The listing builds one solid part. Answer for the finished solid, in the listing's coordinates (mm). A direction names the side the tool comes from. Coordinates: 2 decimals unless noted, no trailing zeros. Order: outer loops, then holes, each group sorted by start corner. A loop starts at its lowest first (then second) coordinate and runs counter-clockwise, first axis right, second up.
```python
from build123d import *

# Parameters (mm, degrees)
SKETCH_W        = 40
SKETCH_H        = 70
SKETCH_R        = 5.5
SKETCH_W_2      = 16
SKETCH_H_2      = 21.5
PAD_DEPTH       = 2
SKETCH001_W     = 5.6
SKETCH001_H     = 5.6
SKETCH001_W_2   = 16
SKETCH001_H_2   = 21.5
PAD001_DEPTH    = 6.5
SKETCH002_R     = 1.625
PAD002_DEPTH    = 2.5
SKETCH003_W     = 16.000008
SKETCH003_H     = 1
SKETCH003_W_2   = 18
POCKET_DEPTH    = 1.5
SKETCH004_W     = 5.3
SKETCH004_H     = 4.3
POCKET001_DEPTH = 2.001
SKETCH005_R     = 1.6
SKETCH005_W     = 8.4
SKETCH005_H     = 1
PAD003_DEPTH    = 1.75
SKETCH006_W     = 36
SKETCH006_H     = 66
SKETCH006_W_2   = 34.4
SKETCH006_H_2   = 64.4
PAD004_DEPTH    = 2.5


with BuildPart() as part:
    # Sketch → Pad (new body)
    with BuildSketch(Plane.XY):
        with Locations((0, -2.25)):
            Rectangle(SKETCH_W, SKETCH_H)
        with Locations((0, 20.75)):
            Circle(SKETCH_R, mode=Mode.SUBTRACT)
        Rectangle(SKETCH_W_2, SKETCH_H_2, mode=Mode.SUBTRACT)
    extrude(amount=PAD_DEPTH)

    # Sketch001 (on Face11 of Pad) → Pad001 (join)
    with BuildSketch(Plane.XY.offset(2)):
        with Locations((-8.5, -18.75)):
            Rectangle(SKETCH001_W, SKETCH001_H)
        with Locations((8.5, -18.75)):
            Rectangle(SKETCH001_W, SKETCH001_H)
        with BuildLine():
            Line((-8, -11.75), (8, -11.75))
            ThreePointArc((9, -10.75), (8.707107, -11.457107), (8, -11.75))
            Line((9, -10.75), (9, 10.75))
            ThreePointArc((8, 11.75), (8.707107, 11.457107), (9, 10.75))
            Line((8, 11.75), (0.8, 11.75))
            ThreePointArc((0.8, 11.75), (0, 14.243313), (-0.8, 11.75))
            Line((-0.8, 11.75), (-8.000008, 11.75))
            ThreePointArc((-9, 10.75), (-8.707109, 11.457104), (-8.000008, 11.75))
            Line((-9, 10.75), (-9, -10.75))
            ThreePointArc((-8, -11.75), (-8.707107, -11.457107), (-9, -10.75))
        make_face()
        Rectangle(SKETCH001_W_2, SKETCH001_H_2, mode=Mode.SUBTRACT)
    extrude(amount=PAD001_DEPTH)

    # Sketch002 (on Face34 of Pad001) → Pad002 (join)
    with BuildSketch(Plane.XY.offset(8.5)):
        with Locations((-8.5, -18.75)):
            Circle(SKETCH002_R)
        with Locations((8.5, -18.75)):
            Circle(SKETCH002_R)
    extrude(amount=PAD002_DEPTH)

    # Sketch003 (on Face35 of Pad002) → Pocket (cut)
    with BuildSketch(Plane.XY.offset(8.5)):
        with Locations((-4e-06, 11.25)):
            Rectangle(SKETCH003_W, SKETCH003_H)
        with Locations((0, -11.25)):
            Rectangle(SKETCH003_W_2, SKETCH003_H)
    extrude(amount=-POCKET_DEPTH, mode=Mode.SUBTRACT)

    # Sketch004 (on Face5 of Pocket) → Pocket001 (cut, through all)
    with BuildSketch(Plane.XY.offset(2)):
        with Locations((12, 20.75)):
            Rectangle(SKETCH004_W, SKETCH004_H)
    extrude(amount=-POCKET001_DEPTH, mode=Mode.SUBTRACT)

    # Sketch005 (on Face5 of Pocket001) → Pad003 (join)
    with BuildSketch(Plane.XY.offset(2)):
        with Locations((12, 15.6)):
            Circle(SKETCH005_R)
        with Locations((12, 12.5)):
            Rectangle(SKETCH005_W, SKETCH005_H)
    extrude(amount=PAD003_DEPTH)

    # Sketch006 (on Face5 of Pad003) → Pad004 (join)
    with BuildSketch(Plane.XY.offset(2)):
        with Locations((0, -2.25)):
            Rectangle(SKETCH006_W, SKETCH006_H)
        with Locations((0, -2.25)):
            Rectangle(SKETCH006_W_2, SKETCH006_H_2, mode=Mode.SUBTRACT)
    extrude(amount=PAD004_DEPTH)


solid = part.part
```
(1) The mould has two halves that part along X. Classify faces 1 (the face through (0, -35.25, 3)), 2 (the face through (0, -10.75, 3)), 3 (the face through (17.2, -3, 3)), 4 (the face through (20, -3, 1)): released by +X, released by -X, zero draft, split by the parting line, or undercut.
(2) Find section B-B (x = 12). Write down the section's boundary in (y, z), and give its area (3 significant figures).
(3) Find section C-C (x = 0). Write down the section's boundary in (y, z).
(4) Find section D-D (y = -18.75). Write down the section's boundary in (x, z) (3 decimals).
(5) Consider line 1 (Y direction, x = 0, z = 0.5); line 2 (X direction, y = -9.5, z = 7.25); line 3 (X direction, y = -4, z = 0.5). Determine where each line is inside the solid, lowest interval first.
(6) For faces 5 (the face through (9.35, 21, 1)), 6 (the face through (18, -3, 3)), 7 (the face through (-18, -3, 3)), 8 (the face through (0, 29.95, 3)), 9 (the face through (0, 32.75, 1)), determine the directions among +Z, -Z, +X, -X, +Y, -Y from which every point of the face is accessible in a straight line to the end or side of a thin tool.
(7) Find section A-A (y = 20.75). Write down the section's boundary in (x, z).
(8) Each of these flat-tipped pins is pushed along its axis until it touches: pin 1 Ø0.8 at (y, z) = (12.5, 3) entering from -X; pin 2 Ø0.9 at (x, z) = (12.5, 2.5) entering from -Y; pin 3 Ø6 at (y, z) = (16, 8) entering from -X. Where does it stop, or does it pass through?
Findings below:
1. face 1: zero draft
1. face 2: undercut
1. face 3: undercut
1. face 4: released by +X
2. outline: (-37.25, 0) - (18.6, 0) - (18.6, 2) - (17.2, 2) - (17.2, 3.75) - (14, 3.75) - (14, 2) - (13, 2) - (13, 3.75) - (12, 3.75) - (12, 2) - (-34.45, 2) - (-34.45, 4.5) - (-35.25, 4.5) - (-35.25, 2) - (-37.25, 2) - close; (22.9, 0) - (32.75, 0) - (32.75, 2) - (30.75, 2) - (30.75, 4.5) - (29.95, 4.5) - (29.95, 2) - (22.9, 2) - close
2. area: 143 mm2
3. outline: (-37.25, 0) - (-10.75, 0) - (-10.75, 7) - (-11.75, 7) - (-11.75, 2) - (-34.45, 2) - (-34.45, 4.5) - (-35.25, 4.5) - (-35.25, 2) - (-37.25, 2) - close; (10.75, 0) - (15.25, 0) - (15.25, 2) - (14.24, 2) - (14.24, 8.5) - (11.75, 8.5) - (11.75, 7) - (10.75, 7) - close; (26.25, 0) - (32.75, 0) - (32.75, 2) - (30.75, 2) - (30.75, 4.5) - (29.95, 4.5) - (29.95, 2) - (26.25, 2) - close
4. outline: (-20, 0) - (20, 0) - (20, 2) - (18, 2) - (18, 4.5) - (17.2, 4.5) - (17.2, 2) - (11.3, 2) - (11.3, 8.5) - (10.125, 8.5) - (10.125, 11) - (6.875, 11) - (6.875, 8.5) - (5.7, 8.5) - (5.7, 2) - (-5.7, 2) - (-5.7, 8.5) - (-6.875, 8.5) - (-6.875, 11) - (-10.125, 11) - (-10.125, 8.5) - (-11.3, 8.5) - (-11.3, 2) - (-17.2, 2) - (-17.2, 4.5) - (-18, 4.5) - (-18, 2) - (-20, 2) - close
5. line 1: y = -37.25 to -10.75, 10.75 to 15.25, 26.25 to 32.75
5. line 2: x = -9 to -8, 8 to 9
5. line 3: x = -20 to -8, 8 to 20
6. face 5: +Z, -Z
6. face 6: +Z, +X, +Y, -Y
6. face 7: +Z, -X, +Y, -Y
6. face 8: +Z
6. face 9: +Z, -Z, +X, -X, +Y
7. outline: (-20, 0) - (-5.5, 0) - (-5.5, 2) - (-17.2, 2) - (-17.2, 4.5) - (-18, 4.5) - (-18, 2) - (-20, 2) - close; (5.5, 0) - (9.35, 0) - (9.35, 2) - (5.5, 2) - close; (14.65, 0) - (20, 0) - (20, 2) - (18, 2) - (18, 4.5) - (17.2, 4.5) - (17.2, 2) - (14.65, 2) - close
8. pin 1: stops at x = -18
8. pin 2: stops at y = -35.25
8. pin 3: stops at x = -1.37
